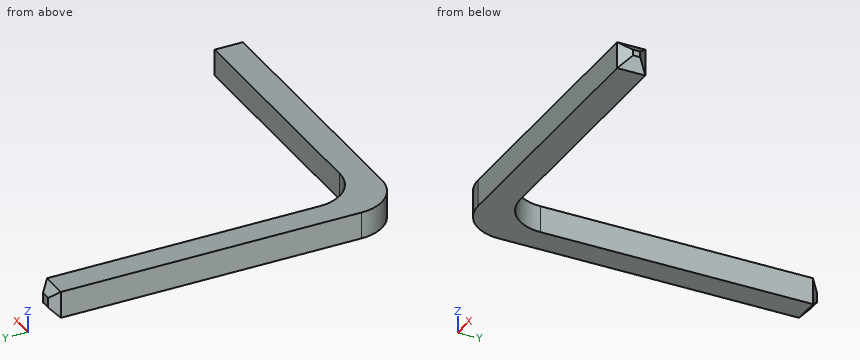
```python
from build123d import *

# Parameters (mm, degrees)
PIN_DRAWING_W       = 0.636
PIN_DRAWING_H       = 0.636
PIN_DEPTH           = 11.54
CHAMFER2_SIZE       = 0.2
SKETCH1_W           = 7
SKETCH1_H           = 0.67
BOSS_EXTRUDE1_DEPTH = 0.636
CHAMFER3_SIZE       = 0.25
SKETCH2_W           = 0.636
SKETCH2_H           = 3.640361057
CUT_EXTRUDE1_DEPTH  = 0.636
FILLET1_R           = 1


with BuildPart() as part:
    # pin_drawing → pin (new body)
    with BuildSketch(Plane(origin=(0, 0, 0), x_dir=(1, 0, 0), z_dir=(0, 1, 0))):
        with Locations((0.318, -0.318)):
            Rectangle(PIN_DRAWING_W, PIN_DRAWING_H)
    extrude(amount=PIN_DEPTH)

    # Chamfer2
    chamfer2_edges = [part.edges().sort_by_distance(p)[0] for p in [
        (0.636, 11.54, 0.318),
        (0.318, 11.54, 0),
        (0, 11.54, 0.318),
        (0.318, 0, 0),
        (0.636, 0, 0.318),
        (0.318, 0, 0.636),
        (0, 0, 0.318),
        (0.318, 11.54, 0.636),
    ]]
    chamfer(chamfer2_edges, length=CHAMFER2_SIZE)

    # Sketch1 → Boss-Extrude1 (add)
    with BuildSketch(Plane(origin=(0, 0, 0), x_dir=(-1, 0, 0), z_dir=(0, 0, -1))):
        with Locations((-4.136, 3.542089627)):
            Rectangle(SKETCH1_W, SKETCH1_H)
    extrude(amount=-BOSS_EXTRUDE1_DEPTH)

    # Chamfer3
    chamfer3_edges = [part.edges().sort_by_distance(p)[0] for p in [
        (7.636, 3.877089627, 0.318),
        (7.636, 3.542089627, 0.636),
        (7.636, 3.542089627, 0),
        (7.636, 3.207089627, 0.318),
    ]]
    chamfer(chamfer3_edges, length=CHAMFER3_SIZE)

    # Sketch2 → Cut-Extrude1 (cut)
    with BuildSketch(Plane(origin=(0, 0, 0), x_dir=(-1, 0, 0), z_dir=(0, 0, -1))):
        with Locations((-0.318, 1.386909099)):
            Rectangle(SKETCH2_W, SKETCH2_H)
    extrude(amount=-CUT_EXTRUDE1_DEPTH, mode=Mode.SUBTRACT)

    # Fillet1
    fillet1_edges = [part.edges().sort_by_distance(p)[0] for p in [
        (0.636, 3.877089627, 0.318),
        (0, 3.207089627, 0.318),
    ]]
    fillet(fillet1_edges, radius=FILLET1_R)


solid = part.part
```
Part model, mm, in its own coordinate system. Round coordinates to 2 decimals unless told otherwise and drop trailing zeros. Write each loop counter-clockwise with the first axis right and the second up, starting at its lowest first coordinate (ties: lowest second). Pieces come first, ordered by that corner, then holes. Notation, with made-up numbers: M 74,-22 L 114,-22 A25 cw 114,7 Z; hole C 66.25,16.25 d8. An arc over 180 degrees is marked long. One line per question, with ' | ' between items.
(1) Saw through at A-A on x = 2.75. Write the cut outline in (y, z).
Answer key:
outline: M 3.21,0 L 3.88,0 L 3.88,0.64 L 3.21,0.64 Z
(2) Probe line 1 along X through (y, z) = (9.25, 0.4); line 2 along Y through (x, z) = (6.5, 0.5); line 3 along Y through (x, z) = (0.5, 0.35). List the from-to ranges inside material, lowest first.
Answer key:
line 1: x = 0 to 0.64 | line 2: y = 3.21 to 3.88 | line 3: y = 3.34 to 11.48
(3) Saw through at B-B on y = 5.5. Write the cut outline in (x, z), then the cut area to 3 significant figures.
Answer key:
outline: M 0,0 L 0.64,0 L 0.64,0.64 L 0,0.64 Z | area: 0.404 mm^2
